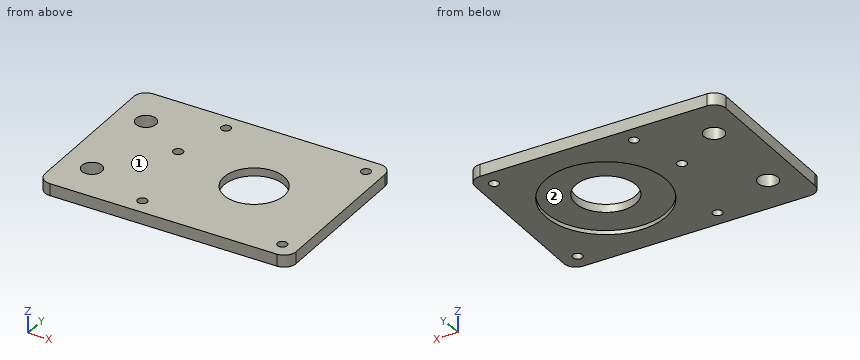
Autodesk Inventor part; units mm, degrees
ref_plane "YZ Plane" through (0, 0, 0) normal (1, 0, 0) x (0, 1, 0)
ref_plane "XZ Plane" through (0, 0, 0) normal (0, 1, 0) x (-1, 0, 0)
ref_plane "XY Plane" through (0, 0, 0) normal (0, 0, 1) x (1, 0, 0)
ref_plane "Płaszczyzna konstrukcyjna1" through (4586.1519, -9.817, 0) normal (0, 0, 1) x (0.999, 0.0439, 0)
sketch "Szkic1" plane through (4586.1519, -9.817, 0) normal (0, 0, 1) x (0.999, 0.0439, 0)
  circle A0 centre (85, 0) radius 5
  circle A1 centre (85, -45) radius 5
  line L0 (76, 21) -> (189, 21)
  line L1 (195, 15) -> (195, -59)
  line L2 (189, -65) -> (76, -65)
  line L3 (70, -59) -> (70, 15)
  arc A2 (70, -59) -> (76, -65) centre (76, -59) ccw
  arc A3 (76, 21) -> (70, 15) centre (76, 15) ccw
  arc A4 (189, -65) -> (195, -59) centre (189, -59) ccw
  arc A5 (195, 15) -> (189, 21) centre (189, 15) ccw
  circle A6 centre (152, -22) radius 30
  circle A7 centre (152, -22) radius 15
  line L4 (117.2, 12.8) -> (186.8, -56.8) construction
  line L5 (186.8, 12.8) -> (117.2, -56.8) construction
  circle A8 centre (117.2, 12.8) radius 2.4
  circle A9 centre (117.2, -56.8) radius 2.4
  circle A10 centre (186.8, -56.8) radius 2.4
  circle A11 centre (186.8, 12.8) radius 2.4
  point P0 (-4581.2965, 211.2059)
  point P1 (195, -65)
  point P2 (195, 21)
  point P3 (70, -65)
  dimension "d0" = 10
  dimension "d1" = 10
  dimension "d2" = 125
  dimension "d3" = 86
  dimension "d4" = 6
  dimension "d7" = 45
  dimension "d8" = 60
  dimension "d9" = 30
  dimension "d10" = 69.6
  dimension "d11" = 69.6
  dimension "d12" = 4.8
  dimension "d13" = 4.8
  dimension "d14" = 4.8
  dimension "d15" = 4.8
extrude "Wyciągnięcie proste1" add sketch "Szkic1" along normal blind 6 contours L0 A5 L1 A4 L2 A2 L3 A3 | A6
extrude "Wyciągnięcie proste2" cut sketch "Szkic1" along normal blind 2 contours A6
thread "Gwint1"
thread "Gwint2"
thread "Gwint3"
thread "Gwint4"
sketch "Szkic3" plane through (4586.1519, -9.817, 0) normal (0, 0, -1) x (-0.999, -0.0439, 0)
  point P0 (-109.5, -14.2897)
hole "Otwór2" at (4696.1738, -19.2843, 0) direction (0, 0, 1) diameter 4.917 end through all
properties part number "mocowanie silnika" material "Tytan"
Geometry check sheet. Reference: the model listing, model coordinates, mm. Face numbers are marked on the shaded views. Round coordinates to 2 decimals unless told otherwise and drop trailing zeros. Loops run counter-clockwise (first coordinate to the right, second up) from the corner with the lowest first, then second, coordinate; pieces in that order, holes last. Notation, with made-up numbers: (27.25, 45.5) - (39.25, 45.5) arc R35 cw to (39.25, 82.5) - close; hole circle Ø2 at (38.5, 27). An arc over 180 degrees is marked (long way). Use a Markdown table: item, result.
Q1. Cross-section at B-B on y = -4. Record the cut outline in (x, z), plus the area to 3 significant figures.
Solutions:
| item | result |
|---|---|
| outline | (4655.96, 0) - (4666.53, 0) - (4666.53, 6) - (4655.96, 6) - close; (4675.61, 0) - (4717.67, 0) - (4717.67, 2) - (4760.27, 2) - (4760.27, 0) - (4781.08, 0) - (4781.08, 6) - (4675.61, 6) - close |
| area | 611 mm2 |
Q2. Go/stop test with flat-tipped pins: P1, Ø18, axis at x = 4727, y = -12, coming from the -Z side; P2, Ø3, axis at y = -13.5, z = 1.5, coming from the +X side; P3, Ø1.5, axis at y = -10, z = 1.5, coming from the -X side. Record where each tip stops, or that it passes through.
Solutions:
| item | result |
|---|---|
| P1 | stops at z = 2 |
| P2 | stops at x = 4781.57 |
| P3 | stops at x = 4656.19 |
Q3. Cross-section at D-D on y = -19. Record the cut outline in (x, z), plus the area to 3 significant figures.
Solutions:
| item | result |
|---|---|
| outline | (4656.62, 0) - (4693.73, 0) - (4693.73, 6) - (4656.62, 6) - close; (4698.62, 0) - (4709.6, 0) - (4709.6, 2) - (4725.28, 2) - (4725.28, 6) - (4698.62, 6) - close; (4752.66, 2) - (4768.34, 2) - (4768.34, 0) - (4781.74, 0) - (4781.74, 6) - (4752.66, 6) - close |
| area | 494 mm2 |
Q4. Material ranges on line 1 (X direction, y = 10, z = 0.75); line 2 (X direction, y = -21, z = 3.1); line 3 (Y direction, x = 4751.5, z = 2.85), recorded low to high.
Solutions:
| item | result |
|---|---|
| line 1 | x = 4655.61 to 4701.19, 4704.16 to 4770.12, 4774.3 to 4780.47 |
| line 2 | x = 4656.71 to 4694.41, 4697.93 to 4724.55, 4753.39 to 4781.83 |
| line 3 | y = -67.61 to -33.37, -16.87 to 18.47 |
Q5. Cross-section at A-A on x = 4737. Record the cut outline in (y, z).
Solutions:
| item | result |
|---|---|
| outline | (-68.25, 0) - (-55.06, 0) - (-55.06, 2) - (-39.99, 2) - (-39.99, 6) - (-68.25, 6) - close; (-10.25, 2) - (4.81, 2) - (4.81, 0) - (17.83, 0) - (17.83, 6) - (-10.25, 6) - close |
Q6. Draft check along X on the marked faces 1 and 2. Enter one of: released by +X, released by -X, zero draft, split by the parting line, or undercut.
Solutions:
| item | result |
|---|---|
| face 1 | zero draft |
| face 2 | undercut |
